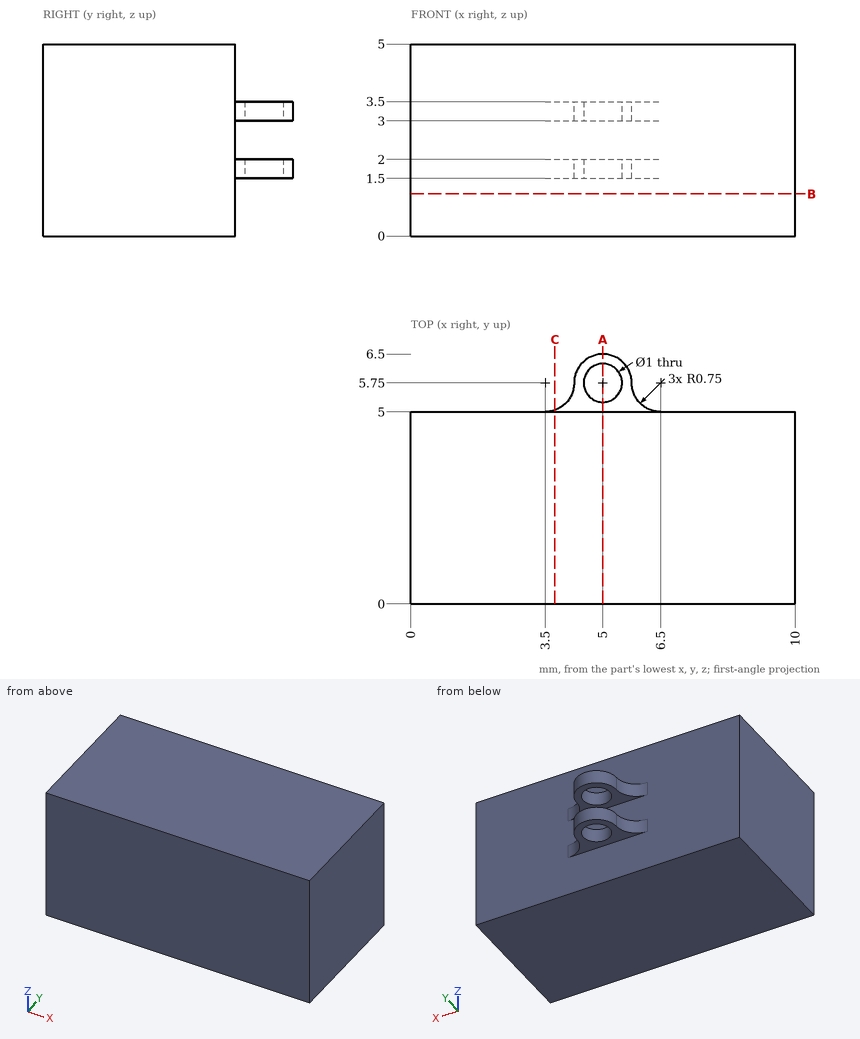
Geometry: see drawing. Coordinates: mm, zero at the bounding-box minimum. Round coordinates to 2 decimals unless told otherwise and drop trailing zeros. Loops run counter-clockwise (first coordinate to the right, second up) from the corner with the lowest first, then second, coordinate; pieces in that order, holes last.
(1) Material intervals for probe 1 along Y at (x, z) = (5, 1.85); probe 2 along Y at (x, z) = (3.5, 4.5); probe 3 along Z at (x, y) = (4.25, 5.25), sorted ascending.
From the geometry:
probe 1: y = 0 to 5.25, 6.25 to 6.5
probe 2: y = 0 to 5
probe 3: z = 1.5 to 2, 3 to 3.5
(2) Section query C-C (x = 3.75). Output: boundary loops of the cut face in (y, z).
From the geometry:
outline: (0, 0) - (5, 0) - (5, 1.5) - (5.04, 1.5) - (5.04, 2) - (5, 2) - (5, 3) - (5.04, 3) - (5.04, 3.5) - (5, 3.5) - (5, 5) - (0, 5) - close
(3) Section query A-A (x = 5). Output: boundary loops of the cut face in (y, z).
From the geometry:
outline: (0, 0) - (5, 0) - (5, 1.5) - (5.25, 1.5) - (5.25, 2) - (5, 2) - (5, 3) - (5.25, 3) - (5.25, 3.5) - (5, 3.5) - (5, 5) - (0, 5) - close; (6.25, 1.5) - (6.5, 1.5) - (6.5, 2) - (6.25, 2) - close; (6.25, 3) - (6.5, 3) - (6.5, 3.5) - (6.25, 3.5) - close
(4) Section query B-B (z = 1.1). Output: boundary loops of the cut face in (x, y), and give its area (3 significant figures).
From the geometry:
outline: (0, 0) - (10, 0) - (10, 5) - (0, 5) - close
area: 50.0 mm2
(5) Contact query for flat-ended pins moving along their axis: pin 1 Ø1 at (x, z) = (3, 4.5) entering from +Y; pin 2 Ø1.6 at (x, y) = (5, 6) entering from -Z; pin 3 Ø1.6 at (x, y) = (5.5, 6) entering from +Z. Output: stop coordinate, or through.
From the geometry:
pin 1: stops at y = 5
pin 2: stops at z = 1.5
pin 3: stops at z = 3.5
